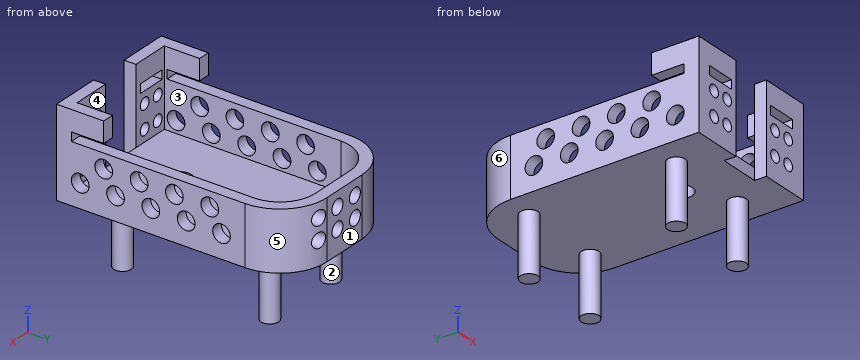
from build123d import *

# Parameters (mm, degrees)
ESQUISSE1_W             = 24
ESQUISSE1_H             = 40
BOSS_EXTRU_1_DEPTH      = 10
CONG_1_R                = 8
COQUE1_T                = -2
ESQUISSE2_W             = 7
ESQUISSE2_H             = 10
ENL_V_MAT_EXTRU_1_DEPTH = 2
ESQUISSE3_R             = 1.5
ENL_V_MAT_EXTRU_2_DEPTH = 33.802438934
ESQUISSE4_R             = 1.25
ENL_V_MAT_EXTRU_3_DEPTH = 13
ENL_V_MAT_EXTRU_4_REACH = 44.942
ESQUISSE5_R             = 1
BOSS_EXTRU_2_DEPTH      = 5
BOSS_EXTRU_2_DEPTH_BACK = 0.5
ENL_V_MAT_EXTRU_5_REACH = 36.655
ESQUISSE8_W             = 1.5
ESQUISSE8_H             = 5.5
ENL_V_MAT_EXTRU_6_REACH = 46.373
ESQUISSE9_W             = 5
ESQUISSE9_H             = 1.5
ENL_V_MAT_EXTRU_7_REACH = 28.702
ESQUISSE10_R            = 2
ESQUISSE11_R            = 1.5
BOSS_EXTRU_3_DEPTH      = 10


with BuildPart() as part:
    # Esquisse1 → Boss.-Extru.1 (new body)
    with BuildSketch(Plane.XY):
        Rectangle(ESQUISSE1_W, ESQUISSE1_H)
    extrude(amount=BOSS_EXTRU_1_DEPTH)

    # Congé1
    cong_1_edges = [part.edges().sort_by_distance(p)[0] for p in [
        (-12, 20, 5),
        (12, 20, 5),
    ]]
    fillet(cong_1_edges, radius=CONG_1_R)

    # Coque1
    coque1_openings = [part.faces().sort_by_distance(p)[0] for p in [
        (0, -0.536491662, 10),
    ]]
    offset(amount=COQUE1_T, openings=coque1_openings, kind=Kind.INTERSECTION)

    # Esquisse2 → Enlèv. mat.-Extru.1 (cut)
    with BuildSketch(Plane.XZ.offset(20)):
        with Locations((0, 5)):
            Rectangle(ESQUISSE2_W, ESQUISSE2_H)
    extrude(amount=-ENL_V_MAT_EXTRU_1_DEPTH, mode=Mode.SUBTRACT)

    # Esquisse3 → Enlèv. mat.-Extru.2 (cut, through all)
    with BuildSketch(Plane(origin=(12, 0, 0), x_dir=(0, 0, -1), z_dir=(1, 0, 0))):
        with Locations(Location((-4, -16, 0), (0, 0, 90))):
            Circle(ESQUISSE3_R)
        with Locations(Location((-7.5, -12, 0), (0, 0, 90))):
            Circle(ESQUISSE3_R)
        with Locations(Location((-7.5, -6, 0), (0, 0, 90))):
            Circle(ESQUISSE3_R)
        with Locations(Location((-4, -10, 0), (0, 0, 90))):
            Circle(ESQUISSE3_R)
        with Locations(Location((-7.5, 0, 0), (0, 0, 90))):
            Circle(ESQUISSE3_R)
        with Locations(Location((-4, -4, 0), (0, 0, 90))):
            Circle(ESQUISSE3_R)
        with Locations(Location((-7.5, 6, 0), (0, 0, 90))):
            Circle(ESQUISSE3_R)
        with Locations(Location((-4, 2, 0), (0, 0, 90))):
            Circle(ESQUISSE3_R)
        with Locations(Location((-4, 8, 0), (0, 0, 90))):
            Circle(ESQUISSE3_R)
    extrude(amount=-ENL_V_MAT_EXTRU_2_DEPTH, mode=Mode.SUBTRACT)

    # Esquisse4 → Enlèv. mat.-Extru.3 (cut)
    with BuildSketch(Plane(origin=(0, 20, 0), x_dir=(1, 0, 0), z_dir=(0, 1, 0))):
        with Locations(Location((-2.4, -4, 0), (0, 0, 270))):
            Circle(ESQUISSE4_R)
        with Locations(Location((1.6, -4, 0), (0, 0, 270))):
            Circle(ESQUISSE4_R)
        with Locations(Location((5.6, -4, 0), (0, 0, 270))):
            Circle(ESQUISSE4_R)
        with Locations(Location((1.6, -7.5, 0), (0, 0, 270))):
            Circle(ESQUISSE4_R)
        with Locations(Location((5.6, -7.5, 0), (0, 0, 270))):
            Circle(ESQUISSE4_R)
        with Locations(Location((-2.4, -7.5, 0), (0, 0, 270))):
            Circle(ESQUISSE4_R)
    extrude(amount=-ENL_V_MAT_EXTRU_3_DEPTH, mode=Mode.SUBTRACT)

    # Esquisse5 → Enlèv. mat.-Extru.4 (cut, up to next)
    with BuildSketch(Plane.XZ.offset(20), mode=Mode.PRIVATE) as enl_v_mat_extru_4_sk1:
        with Locations(Location((-8.5, 8, 0), (0, 0, 270))):
            Circle(ESQUISSE5_R)
    enl_v_mat_extru_4_tool1 = extrude(enl_v_mat_extru_4_sk1.sketch, amount=-ENL_V_MAT_EXTRU_4_REACH, mode=Mode.PRIVATE) & part.part
    # Esquisse5 → Enlèv. mat.-Extru.4 (cut, up to next)
    with BuildSketch(Plane.XZ.offset(20), mode=Mode.PRIVATE) as enl_v_mat_extru_4_sk2:
        with Locations(Location((-5.5, 8, 0), (0, 0, 270))):
            Circle(ESQUISSE5_R)
    enl_v_mat_extru_4_tool2 = extrude(enl_v_mat_extru_4_sk2.sketch, amount=-ENL_V_MAT_EXTRU_4_REACH, mode=Mode.PRIVATE) & part.part
    # Esquisse5 → Enlèv. mat.-Extru.4 (cut, up to next)
    with BuildSketch(Plane.XZ.offset(20), mode=Mode.PRIVATE) as enl_v_mat_extru_4_sk3:
        with Locations(Location((-5.5, 4, 0), (0, 0, 270))):
            Circle(ESQUISSE5_R)
    enl_v_mat_extru_4_tool3 = extrude(enl_v_mat_extru_4_sk3.sketch, amount=-ENL_V_MAT_EXTRU_4_REACH, mode=Mode.PRIVATE) & part.part
    # Esquisse5 → Enlèv. mat.-Extru.4 (cut, up to next)
    with BuildSketch(Plane.XZ.offset(20), mode=Mode.PRIVATE) as enl_v_mat_extru_4_sk4:
        with Locations(Location((-8.5, 4, 0), (0, 0, 270))):
            Circle(ESQUISSE5_R)
    enl_v_mat_extru_4_tool4 = extrude(enl_v_mat_extru_4_sk4.sketch, amount=-ENL_V_MAT_EXTRU_4_REACH, mode=Mode.PRIVATE) & part.part
    # Esquisse5 → Enlèv. mat.-Extru.4 (cut, up to next)
    with BuildSketch(Plane.XZ.offset(20), mode=Mode.PRIVATE) as enl_v_mat_extru_4_sk5:
        with Locations(Location((8.5, 4, 0), (0, 0, 90))):
            Circle(ESQUISSE5_R)
    enl_v_mat_extru_4_tool5 = extrude(enl_v_mat_extru_4_sk5.sketch, amount=-ENL_V_MAT_EXTRU_4_REACH, mode=Mode.PRIVATE) & part.part
    # Esquisse5 → Enlèv. mat.-Extru.4 (cut, up to next)
    with BuildSketch(Plane.XZ.offset(20), mode=Mode.PRIVATE) as enl_v_mat_extru_4_sk6:
        with Locations(Location((5.5, 4, 0), (0, 0, 90))):
            Circle(ESQUISSE5_R)
    enl_v_mat_extru_4_tool6 = extrude(enl_v_mat_extru_4_sk6.sketch, amount=-ENL_V_MAT_EXTRU_4_REACH, mode=Mode.PRIVATE) & part.part
    # Esquisse5 → Enlèv. mat.-Extru.4 (cut, up to next)
    with BuildSketch(Plane.XZ.offset(20), mode=Mode.PRIVATE) as enl_v_mat_extru_4_sk7:
        with Locations(Location((5.5, 8, 0), (0, 0, 90))):
            Circle(ESQUISSE5_R)
    enl_v_mat_extru_4_tool7 = extrude(enl_v_mat_extru_4_sk7.sketch, amount=-ENL_V_MAT_EXTRU_4_REACH, mode=Mode.PRIVATE) & part.part
    # Esquisse5 → Enlèv. mat.-Extru.4 (cut, up to next)
    with BuildSketch(Plane.XZ.offset(20), mode=Mode.PRIVATE) as enl_v_mat_extru_4_sk8:
        with Locations(Location((8.5, 8, 0), (0, 0, 90))):
            Circle(ESQUISSE5_R)
    enl_v_mat_extru_4_tool8 = extrude(enl_v_mat_extru_4_sk8.sketch, amount=-ENL_V_MAT_EXTRU_4_REACH, mode=Mode.PRIVATE) & part.part
    add(enl_v_mat_extru_4_tool1.solids().sort_by_distance((-8.5, -20, 8))[0], mode=Mode.SUBTRACT)
    add(enl_v_mat_extru_4_tool2.solids().sort_by_distance((-5.5, -20, 8))[0], mode=Mode.SUBTRACT)
    add(enl_v_mat_extru_4_tool3.solids().sort_by_distance((-5.5, -20, 4))[0], mode=Mode.SUBTRACT)
    add(enl_v_mat_extru_4_tool4.solids().sort_by_distance((-8.5, -20, 4))[0], mode=Mode.SUBTRACT)
    add(enl_v_mat_extru_4_tool5.solids().sort_by_distance((8.5, -20, 4))[0], mode=Mode.SUBTRACT)
    add(enl_v_mat_extru_4_tool6.solids().sort_by_distance((5.5, -20, 4))[0], mode=Mode.SUBTRACT)
    add(enl_v_mat_extru_4_tool7.solids().sort_by_distance((5.5, -20, 8))[0], mode=Mode.SUBTRACT)
    add(enl_v_mat_extru_4_tool8.solids().sort_by_distance((8.5, -20, 8))[0], mode=Mode.SUBTRACT)

    # Esquisse7 → Boss.-Extru.2 (add, two sides: drawn at the far end of the back side and taken through both)
    with BuildSketch(Plane.XY.offset(10).offset(-BOSS_EXTRU_2_DEPTH_BACK)):
        Polygon((-12, -12), (-12, -20), (-3.5, -20), (-3.5, -18), (-10, -18), (-10, -12), align=None)
        Polygon((12, -12), (12, -20), (3.5, -20), (3.5, -18), (10, -18), (10, -12), align=None)
    extrude(amount=BOSS_EXTRU_2_DEPTH + BOSS_EXTRU_2_DEPTH_BACK)

    # Esquisse8 → Enlèv. mat.-Extru.5 (cut, up to next)
    with BuildSketch(Plane(origin=(12, 0, 0), x_dir=(0, 0, -1), z_dir=(1, 0, 0)), mode=Mode.PRIVATE) as enl_v_mat_extru_5_sk1:
        with Locations((-10.75, -14.75)):
            Rectangle(ESQUISSE8_W, ESQUISSE8_H)
    enl_v_mat_extru_5_tool1 = extrude(enl_v_mat_extru_5_sk1.sketch, amount=-ENL_V_MAT_EXTRU_5_REACH, mode=Mode.PRIVATE) & part.part
    enl_v_mat_extru_5 = enl_v_mat_extru_5_tool1.solids().sort_by_distance((12, -14.75, 10.75))[0]
    add(enl_v_mat_extru_5, mode=Mode.SUBTRACT)

    # Esquisse9 → Enlèv. mat.-Extru.6 (cut, up to next)
    with BuildSketch(Plane.XZ.offset(20), mode=Mode.PRIVATE) as enl_v_mat_extru_6_sk1:
        with Locations((7, 10.75)):
            Rectangle(ESQUISSE9_W, ESQUISSE9_H)
    enl_v_mat_extru_6_tool1 = extrude(enl_v_mat_extru_6_sk1.sketch, amount=-ENL_V_MAT_EXTRU_6_REACH, mode=Mode.PRIVATE) & part.part
    enl_v_mat_extru_6 = enl_v_mat_extru_6_tool1.solids().sort_by_distance((7, -20, 10.75))[0]
    add(enl_v_mat_extru_6, mode=Mode.SUBTRACT)

    # Symétrie1: Enlèv. mat.-Extru.5, Enlèv. mat.-Extru.6 across plane
    add(enl_v_mat_extru_5.mirror(Plane(origin=(0, 0, 0), x_dir=(0, 0, 1), z_dir=(1, 0, 0))), mode=Mode.SUBTRACT)
    add(enl_v_mat_extru_6.mirror(Plane(origin=(0, 0, 0), x_dir=(0, 0, 1), z_dir=(1, 0, 0))), mode=Mode.SUBTRACT)

    # Esquisse10 → Enlèv. mat.-Extru.7 (cut, up to next)
    with BuildSketch(Plane.XY.offset(2), mode=Mode.PRIVATE) as enl_v_mat_extru_7_sk1:
        with Locations((0, -8)):
            Circle(ESQUISSE10_R)
    enl_v_mat_extru_7_tool1 = extrude(enl_v_mat_extru_7_sk1.sketch, amount=-ENL_V_MAT_EXTRU_7_REACH, mode=Mode.PRIVATE) & part.part
    add(enl_v_mat_extru_7_tool1.solids().sort_by_distance((0, -8, 2))[0], mode=Mode.SUBTRACT)

    # Esquisse11 → Boss.-Extru.3 (add)
    with BuildSketch(Plane(origin=(0, 0, 0), x_dir=(-1, 0, 0), z_dir=(0, 0, -1))):
        with Locations(Location((-7, 12.5, 0), (0, 0, 180))):
            Circle(ESQUISSE11_R)
        with Locations(Location((7, 12.5, 0), (0, 0, 180))):
            Circle(ESQUISSE11_R)
        with Locations(Location((-7, -12.5, 0), (0, 0, 180))):
            Circle(ESQUISSE11_R)
        with Locations(Location((7, -12.5, 0), (0, 0, 180))):
            Circle(ESQUISSE11_R)
    extrude(amount=BOSS_EXTRU_3_DEPTH)


solid = part.part
Check sheet for the modelled part. Datum: model origin and axes. Units: mm. Face numbers are marked on the shaded views. A direction names the side the tool comes from. Round coordinates to 2 decimals unless told otherwise and drop trailing zeros. Order: outer loops, then holes, each group sorted by start corner. A loop starts at its lowest first (then second) coordinate and runs counter-clockwise, first axis right, second up.
(1) Go/stop test with flat-tipped pins: P1, Ø3.5, axis at y = -4, z = 4, coming from the +X side; P2, Ø1.6, axis at x = 7, y = -19.5, coming from the -Z side; P3, Ø10, axis at x = -1, y = -7.5, coming from the +Z side; P4, Ø2.5, axis at x = -8.5, z = 8, coming from the +Y side. Record where each tip stops, or that it passes through.
(2) Cross-section at A-A, the plane y = 8. Enter the section's corners in (x, z).
(3) Access from +Z, -Z, +X, -X, +Y, -Y to the whole of each face (thin tool, end or side, straight path). Record for the marked faces 1, 2 and 3.
(4) Cross-section at B-B, the plane z = -8. Enter the section's corners in (x, y).
(5) Cross-section at D-D, the plane x = 5. Enter the section's corners in (y, z).
(6) Draft check along X on the marked faces 4, 5 and 6. Enter one of: pulls with the +X half, pulls with the -X half, needs draft (parallel to the pull), parting line crosses it, or undercut.
(7) Scan lines: probe 1 along X at (y, z) = (-19, 8); probe 2 along X at (y, z) = (3, 8.5); probe 3 along Z at (x, y) = (-10.5, 0). Record each from-to range of solid material in increasing order.
(8) Cross-section at C-C, the plane x = -5. Enter the section's corners in (y, z).
Check sheet entries:
1. P1: stops at x = 12
1. P2: stops at z = 0
1. P3: stops at z = 2
1. P4: stops at y = 19.31
2. outline: (-12, 0) - (12, 0) - (12, 2.5) - (10, 2.5) - (10, 2) - (-10, 2) - (-10, 2.5) - (-12, 2.5) - close; (-12, 5.5) - (-10, 5.5) - (-10, 10) - (-12, 10) - close; (10, 5.5) - (12, 5.5) - (12, 10) - (10, 10) - close
3. face 1: +Z, -Z, +X, -X, +Y
3. face 2: -Z
3. face 3: +Z
4. outline: circle Ø3 at (-7, -12.5); circle Ø3 at (-7, 12.5); circle Ø3 at (7, -12.5); circle Ø3 at (7, 12.5)
5. outline: (-20, 0) - (19.94, 0) - (19.94, 2.9) - (17.92, 2.9) - (17.92, 2) - (-18, 2) - (-18, 3.13) - (-20, 3.13) - close; (-20, 4.87) - (-18, 4.87) - (-18, 7.13) - (-20, 7.13) - close; (-20, 8.87) - (-18, 8.87) - (-18, 10) - (-20, 10) - close; (-20, 11.5) - (-18, 11.5) - (-18, 15) - (-20, 15) - close; (17.92, 5.1) - (19.94, 5.1) - (19.94, 6.4) - (17.92, 6.4) - close; (17.92, 8.6) - (19.94, 8.6) - (19.94, 10) - (17.92, 10) - close
6. face 4: undercut
6. face 5: pulls with the +X half
6. face 6: pulls with the -X half
7. probe 1: x = -12 to -9.5, -7.5 to -6.5, -4.5 to -3.5, 3.5 to 4.5, 6.5 to 7.5, 9.5 to 12
7. probe 2: x = -12 to -10, 10 to 12
7. probe 3: z = 0 to 6, 9 to 10
8. outline: (-20, 0) - (19.94, 0) - (19.94, 10) - (17.92, 10) - (17.92, 2) - (-18, 2) - (-18, 3.13) - (-20, 3.13) - close; (-20, 4.87) - (-18, 4.87) - (-18, 7.13) - (-20, 7.13) - close; (-20, 8.87) - (-18, 8.87) - (-18, 10) - (-20, 10) - close; (-20, 11.5) - (-18, 11.5) - (-18, 15) - (-20, 15) - close
